Job drawing, mm, ordinate dimensions from the low corner. One solid piece. Give positions to 0.01 mm unless a question says otherwise; leave off trailing zeros. Write each loop counter-clockwise with the first axis right and the second up, starting at its lowest first coordinate (ties: lowest second). Pieces come first, ordered by that corner, then holes. Notation, with made-up numbers: M 5.5,43.25 L 27.5,43.25 A26 cw 27.5,57.25 Z; hole C -33.75,1 d3. An arc over 180 degrees is marked long. Use a Markdown table: item, result.
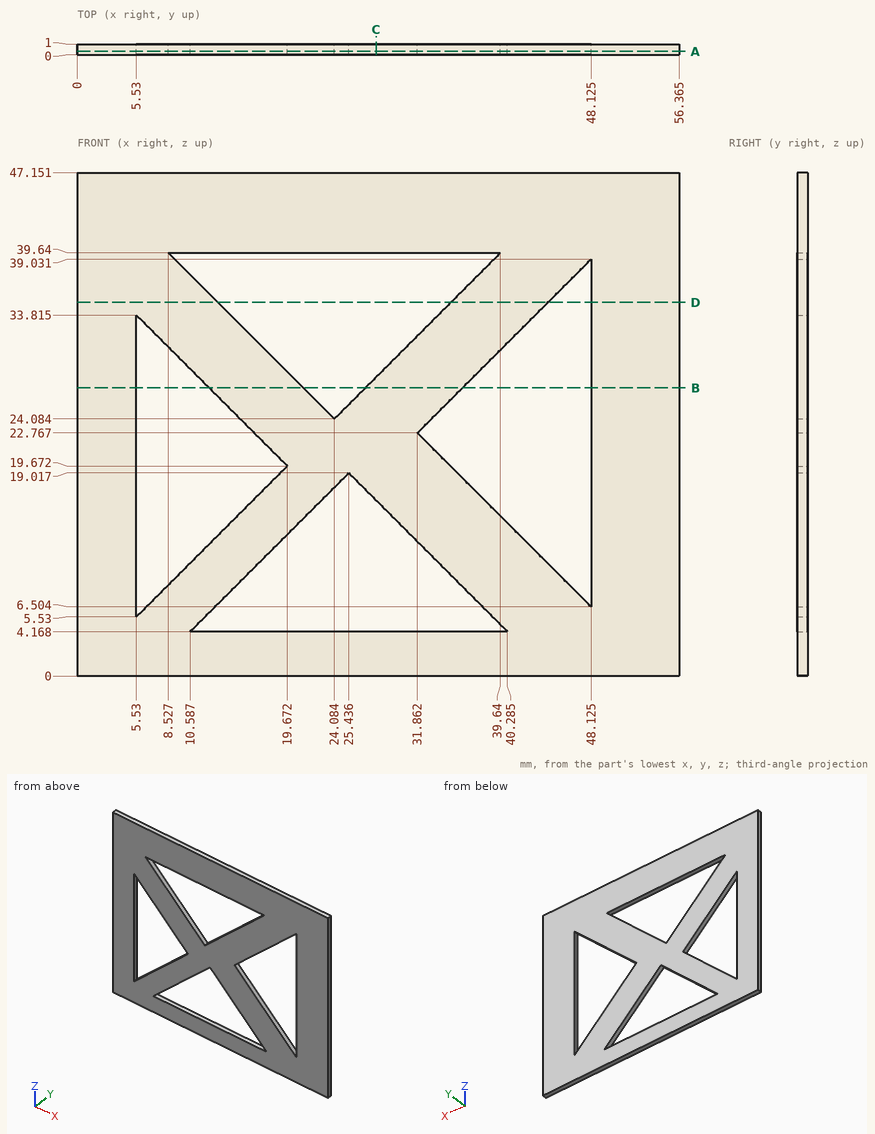
1. Drill centre lines: L1, parallel to X at y = 0.3, z = 11.5 (1 decimal); L2, parallel to X at y = 0.65, z = 26.5 (1 decimal); L3, parallel to Z at x = 24.5, y = 0.7. Where is each one in solid material? Low to high.
Findings below:
| item | result |
|---|---|
| L1 | 0 to 5.5, 11.5 to 17.9, 33 to 43.1, 48.1 to 56.4 |
| L2 | 0 to 5.5, 12.8 to 21.7, 26.5 to 35.6, 48.1 to 56.4 |
| L3 | 0 to 4.17, 18.08 to 24.5, 39.64 to 47.15 |
2. Cut at C-C, the plane x = 28. Give the cut face in (y, z).
Findings below:
| item | result |
|---|---|
| outline | M 0,0 L 1,0 L 1,4.17 L 0,4.17 Z; M 0,16.45 L 1,16.45 L 1,28 L 0,28 Z; M 0,39.64 L 1,39.64 L 1,47.15 L 0,47.15 Z |
3. Cut at B-B, the plane z = 27. Give the cut face in (x, y) (1 decimal).
Findings below:
| item | result |
|---|---|
| outline | M 0,0 L 5.5,0 L 5.5,1 L 0,1 Z; M 12.3,0 L 21.2,0 L 21.2,1 L 12.3,1 Z; M 27,0 L 36.1,0 L 36.1,1 L 27,1 Z; M 48.1,0 L 56.4,0 L 56.4,1 L 48.1,1 Z |
4. Cut at A-A, the plane y = 0.3. State how many separate pieces and enclosed holes the cut face has, then the cut area to 3 significant figures.
Findings below:
| item | result |
|---|---|
| separate pieces | 1 |
| enclosed holes | 4 |
| area | 1,730 mm2 |
5. Cut at D-D, the plane z = 35. Give the cut face in (x, y) (1 decimal).
Findings below:
| item | result |
|---|---|
| outline | M 0,0 L 13.2,0 L 13.2,1 L 0,1 Z; M 35,0 L 44.1,0 L 44.1,1 L 35,1 Z; M 48.1,0 L 56.4,0 L 56.4,1 L 48.1,1 Z |
